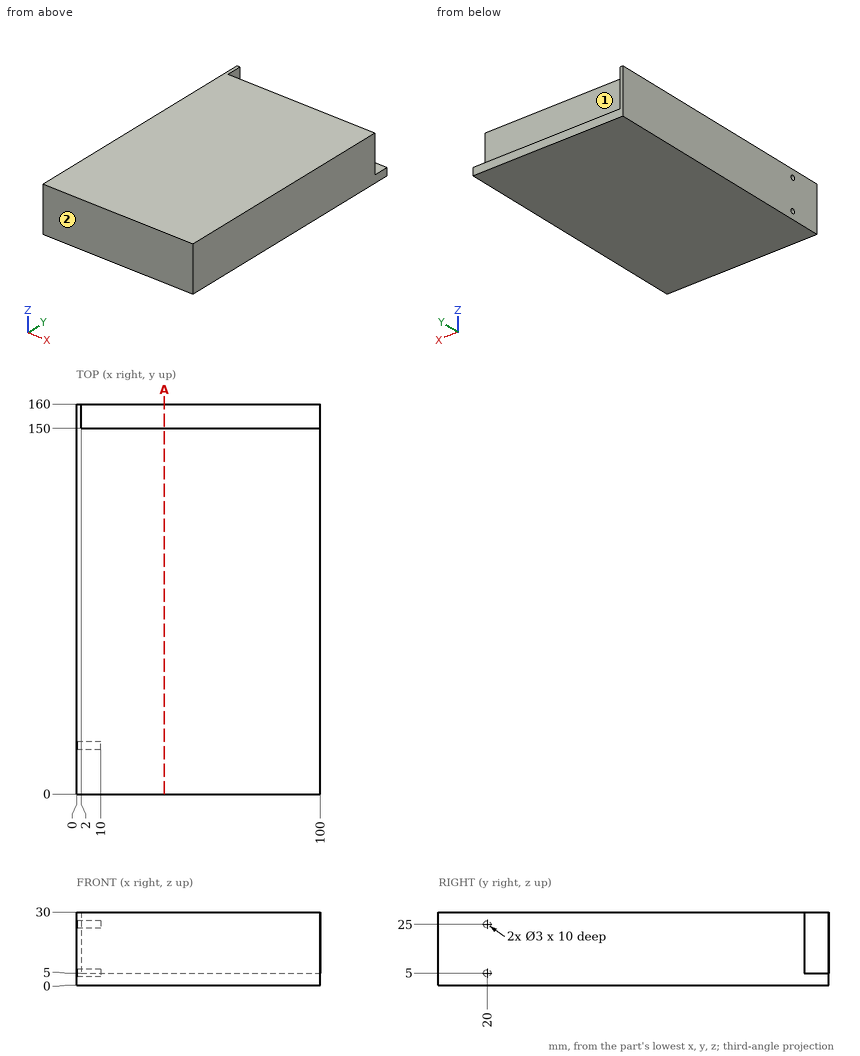
For this review, use the dimensioned drawing (mm, ordinates from the lowest corner) and the shaded views. A direction names the side the tool comes from. Give positions to 0.01 mm unless a question says otherwise; leave off trailing zeros. Order: outer loops, then holes, each group sorted by start corner. A loop starts at its lowest first (then second) coordinate and runs counter-clockwise, first axis right, second up. Notation, with made-up numbers: M -9.5,28 L 37.5,28 A23 ccw 37.5,48 Z; hole C 89.5,-22 d8. An arc over 180 degrees is marked long. One line per question, with ' | ' between items. Start each with the question number.
1) Clearance check with flat-ended pins moving along their axes: P1, Ø2.5, axis at y = 20, z = 5, coming from the -X side; P2, Ø3, axis at x = 59.5, y = 154, coming from the +Z side. State where each tip first meets the part, or that it passes through.
2) For the marked faces 1 and 2, list the 3-axis set-ups (+Z, -Z, +X, -X, +Y, -Y) from which the entire face can be reached by the end or side of a thin tool; tool diameter is ignored.
3) Wall thickness on L1, parallel to Z at x = 2, y = 20; L2, parallel to Y at x = 21, z = 11.75; L3, parallel to X at y = 153, z = 24.75: over which ranges is each line inside the solid? List them lowest first. Write a range as from..to.
4) Consider section A-A, the plane x = 36. Give the boundary of the cut face in (y, z), then the cut area to 3 significant figures.
Found:
1) P1: stops at x = 10 | P2: stops at z = 5
2) face 1: +Z, +X, +Y | face 2: +Z, -Z, +X, -X, -Y
3) L1: z = 0..3.5, 6.5..23.5, 26.5..30 | L2: y = 0..150 | L3: x = 0..2
4) outline: M 0,0 L 160,0 L 160,5 L 150,5 L 150,30 L 0,30 Z | area: 4,550 mm²
